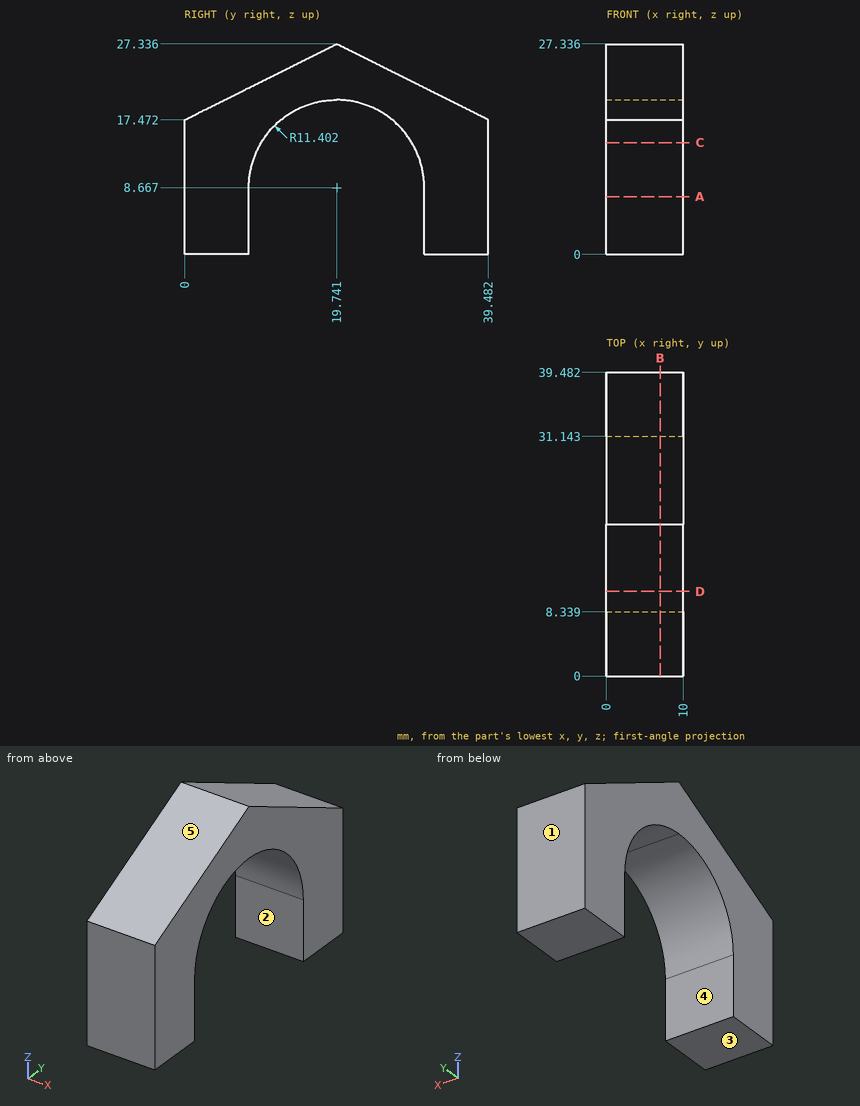
Geometry: see drawing. Coordinates: mm, zero at the bounding-box minimum. A direction names the side the tool comes from. Give positions to 0.01 mm unless a question says otherwise; leave off trailing zeros. Loops run counter-clockwise (first coordinate to the right, second up) from the corner with the lowest first, then second, coordinate; pieces in that order, holes last. Notation, with made-up numbers: (85.5, 19) -> (96.5, 19) arc R24 cw to (96.5, 43) -> close; hole circle Ø7 at (5, 88). An arc over 180 degrees is marked (long way). Put each result on its own line as item: value.
1. Set-up query: the marked faces 1 and 2. Return all of +Z, -Z, +X, -X, +Y, -Y with unobstructed straight access to the full face (end or side cutting, diameter ignored); none if empty.
Taken from the geometry:
face 1: +Z, -Z, +X, -X, +Y
face 2: -Z, +X, -X
2. Pull-direction query (Y, two-part tool) for the marked faces 3, 4 and 5; classes: released by +Y, released by -Y, zero draft, split by the parting line, or undercut.
Taken from the geometry:
face 3: zero draft
face 4: undercut
face 5: released by -Y
3. Cut plane D-D (y = 11). Return the cut outline in (x, z).
Taken from the geometry:
outline: (0, 15.99) -> (10, 15.99) -> (10, 22.97) -> (0, 22.97) -> close
4. Ray query, line 1 along Y through (x, z) = (9.5, 5); line 2 along Y through (x, z) = (4, 18.5) (1 decimal); line 3 along Y through (x, z) = (1, 24.5) (1 decimal). Return the intervals inside material, ascending. Write a range as [from, to].
Taken from the geometry:
line 1: y = [0, 8.34], [31.14, 39.48]
line 2: y = [2.1, 14], [25.5, 37.4]
line 3: y = [14.1, 25.4]
5. Cut plane B-B (x = 7). Return the cut outline in (y, z) (1 decimal).
Taken from the geometry:
outline: (0, 0) -> (8.3, 0) -> (8.3, 8.7) arc R11.4 cw to (31.1, 8.7) -> (31.1, 0) -> (39.5, 0) -> (39.5, 17.5) -> (19.7, 27.3) -> (0, 17.5) -> close
6. Cut plane A-A (z = 7.5). Return the cut outline in (x, y), plus the area to 3 significant figures.
Taken from the geometry:
outline: (0, 0) -> (10, 0) -> (10, 8.34) -> (0, 8.34) -> close; (0, 31.14) -> (10, 31.14) -> (10, 39.48) -> (0, 39.48) -> close
area: 167 mm2
7. Pin query (flat end, axial travel): P1, Ø1, axis at y = 26, z = 17.5, coming from the +X side; P2, Ø3, axis at x = 9, y = 15.5, coming from the -Z side. Return the tip coordinate at first contact, or that it passes through.
Taken from the geometry:
P1: passes through
P2: stops at z = 18.52
8. Cut plane C-C (z = 14.5). Return the cut outline in (x, y) (1 decimal), plus the area to 3 significant figures.
Taken from the geometry:
outline: (0, 0) -> (10, 0) -> (10, 9.9) -> (0, 9.9) -> close; (0, 29.5) -> (10, 29.5) -> (10, 39.5) -> (0, 39.5) -> close
area: 199 mm2
